```python
from build123d import *

# Parameters (mm, degrees)
F0_W     = 65.024
F0_H     = 68.072
F1_DEPTH = 68.072
F2_W     = 65.024
F2_H     = 65.024
F3_DEPTH = 65.024
F4_R     = 19.05
F4_R_2   = 2.794
F5_DEPTH = 3.049
F7_DEPTH = 68.073


with BuildPart() as f1:
    # F0 (on Top) → F1 (new body)
    with BuildSketch(Plane.XY):
        Rectangle(F0_W, F0_H)
    extrude(amount=F1_DEPTH)

    # F2 (on face) → F3 (cut)
    with BuildSketch(Plane.XY.offset(68.072)):
        with Locations((0, 1.524)):
            Rectangle(F2_W, F2_H)
    extrude(amount=-F3_DEPTH, mode=Mode.SUBTRACT)

    # F4 (on face) → F5 (cut, through all)
    with BuildSketch(Plane.XY.offset(3.048)):
        with Locations((0, 5.08)):
            Circle(F4_R)
        with Locations((-23.495, 28.575)):
            Circle(F4_R_2)
        with Locations((23.495, 28.575)):
            Circle(F4_R_2)
        with Locations((23.495, -18.415)):
            Circle(F4_R_2)
        with Locations((-23.495, -18.415)):
            Circle(F4_R_2)
    extrude(amount=-F5_DEPTH, mode=Mode.SUBTRACT)

    # F6 (on face) → F7 (cut, through all)
    with BuildSketch(Plane.XZ.offset(34.036)):
        with BuildLine():
            ThreePointArc((-17.78, 57.912), (-19.939, 60.071), (-22.098, 57.912))
            Line((-22.098, 57.912), (-22.098, 16.256))
            ThreePointArc((-22.098, 16.256), (-19.939, 14.097), (-17.78, 16.256))
            Line((-17.78, 16.256), (-17.78, 57.912))
        make_face()
        with BuildLine():
            ThreePointArc((22.098, 57.912), (19.939, 60.071), (17.78, 57.912))
            Line((17.78, 57.912), (17.78, 16.256))
            ThreePointArc((17.78, 16.256), (19.939, 14.097), (22.098, 16.256))
            Line((22.098, 16.256), (22.098, 57.912))
        make_face()
    extrude(amount=-F7_DEPTH, mode=Mode.SUBTRACT)


solid = f1.part
```
Geometry check sheet. Reference: the model listing, model coordinates, mm. A direction names the side the tool comes from. Give positions to 0.01 mm unless a question says otherwise; leave off trailing zeros. Order: outer loops, then holes, each group sorted by start corner. A loop starts at its lowest first (then second) coordinate and runs counter-clockwise, first axis right, second up.
1. Section check C-C, the plane y = 5.08. Enter the section's corners in (x, z).
2. Section check D-D, the plane x = -24. Enter the section's corners in (y, z).
3. Section check A-A, the plane z = 25. Enter the section's corners in (x, y), and give its area (3 significant figures).
4. Gauge pin test, flat ends, axial feed: pin 1 Ø9 at (x, y) = (-23.495, -18.415) entering from +Z; pin 2 Ø6 at (x, z) = (-19.5, 32.5) entering from +Y; pin 3 Ø1 at (x, y) = (-18, 4.5) entering from -Z. Record the tip position at first contact, or that the pin passes through.
5. Section check B-B, the plane x = 0. Enter the section's corners in (y, z), and give its area (3 significant figures).
6. Access from +Z, -Z, +X, -X, +Y, -Y to the whole of each face (thin tool, end or side, straight path). Record for faces 5 (the face through (-20.83, 29.41, 1.55)), 6 (the face through (-19.89, -32.53, 60.07)), 7 (the face through (0, -30.988, 36)).
7. Release check for a two-part mould opening along Z. For faces 1 (the face through (-22.098, -33, 37)), 2 (the face through (0, -32, 68.072)), 3 (the face through (22.098, -33, 37)), 4 (the face through (0, 34.036, 2)) record: pulls with the +Z half, pulls with the -Z half, needs draft (parallel to the pull), parting line crosses it, or undercut.
8. Thickness scan on L1, parallel to Z at x = 25, y = 6.5; L2, parallel to Y at x = -14, z = 13.5; L3, parallel to Y at x = 0, z = 2.3. Record the ranges inside material, lowest first.
Values follow:
1. outline: (-32.51, 0) - (-19.05, 0) - (-19.05, 3.05) - (-32.51, 3.05) - close; (19.05, 0) - (32.51, 0) - (32.51, 3.05) - (19.05, 3.05) - close
2. outline: (-34.04, 0) - (-21.16, 0) - (-21.16, 3.05) - (-30.99, 3.05) - (-30.99, 68.07) - (-34.04, 68.07) - close; (-15.67, 0) - (25.83, 0) - (25.83, 3.05) - (-15.67, 3.05) - close; (31.32, 0) - (34.04, 0) - (34.04, 3.05) - (31.32, 3.05) - close
3. outline: (-32.51, -34.04) - (-22.1, -34.04) - (-22.1, -30.99) - (-32.51, -30.99) - close; (-17.78, -34.04) - (17.78, -34.04) - (17.78, -30.99) - (-17.78, -30.99) - close; (22.1, -34.04) - (32.51, -34.04) - (32.51, -30.99) - (22.1, -30.99) - close
3. area: 172 mm2
4. pin 1: stops at z = 3.05
4. pin 2: stops at y = -30.99
4. pin 3: passes through
5. outline: (-34.04, 0) - (-13.97, 0) - (-13.97, 3.05) - (-30.99, 3.05) - (-30.99, 68.07) - (-34.04, 68.07) - close; (24.13, 0) - (34.04, 0) - (34.04, 3.05) - (24.13, 3.05) - close
5. area: 290 mm2
6. face 5: +Z, -Z
6. face 6: +Y, -Y
6. face 7: +Z, +X, -X, +Y
7. face 1: undercut
7. face 2: pulls with the +Z half
7. face 3: undercut
7. face 4: needs draft
8. L1: z = 0 to 3.05
8. L2: y = -34.04 to -30.99
8. L3: y = -34.04 to -13.97, 24.13 to 34.04
